For this review, take the finished solid that the model builds, in its own axes (mm). Round coordinates to 2 decimals unless told otherwise and drop trailing zeros. Loops run counter-clockwise (first coordinate to the right, second up) from the corner with the lowest first, then second, coordinate; pieces in that order, holes last. Notation, with made-up numbers: (-13, -7.5) -> (42, -7.5) arc R16 ccw to (42, 11.5) -> close; hole circle Ø9 at (86.5, -24). An arc over 180 degrees is marked (long way). One line per question, with ' | ' between items. Start each with the question number.
1. Consider section A-A (x = -5). Write out the cut boundary in (y, z) (3 decimals).
2. Wall thickness on line 1 along Y through (x, z) = (23, 0.9); line 2 along Y through (x, z) = (36, 1.2) (3 decimals): over which ranges is each line inside the solid? List them lowest first.
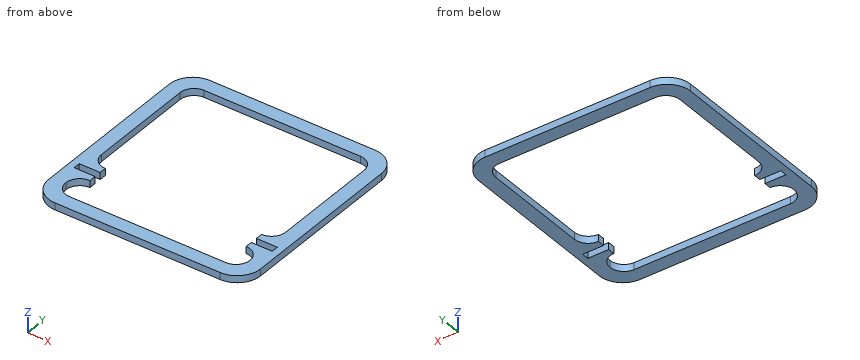
```python
from build123d import *

# Parameters (mm, degrees)
SKETCH1_W           = 96.52
SKETCH1_H           = 96.52
BOSS_EXTRUDE1_DEPTH = 3.175
FILLET1_R           = 10.668
FILLET2_R           = 6.35
FILLET3_R           = 6.35


with BuildPart() as part:
    # Sketch1 → Boss-Extrude1 (new body)
    with BuildSketch(Plane.XY):
        Rectangle(SKETCH1_W, SKETCH1_H)
        Polygon((-41.91, -41.91), (-41.91, -29.21), (-35.56, -29.21), (-35.56, -26.035), (-45.085, -26.035), (-45.085, -22.86), (-35.56, -22.86), (-35.56, -19.685), (-41.91, -19.685), (-41.91, 41.91), (41.91, 41.91), (41.91, -19.685), (35.56, -19.685), (35.56, -22.86), (45.085, -22.86), (45.085, -26.035), (35.56, -26.035), (35.56, -29.21), (41.91, -29.21), (41.91, -41.91), align=None, mode=Mode.SUBTRACT)
    extrude(amount=BOSS_EXTRUDE1_DEPTH)

    # Fillet1
    fillet1_edges = [part.edges().sort_by_distance(p)[0] for p in [
        (48.26, -48.26, 1.5875),
        (-48.26, -48.26, 1.5875),
        (-48.26, 48.26, 1.5875),
        (48.26, 48.26, 1.5875),
    ]]
    fillet(fillet1_edges, radius=FILLET1_R)

    # Fillet2
    fillet2_edges = [part.edges().sort_by_distance(p)[0] for p in [
        (-41.91, -41.91, 1.5875),
        (41.91, -41.91, 1.5875),
        (41.91, 41.91, 1.5875),
        (-41.91, 41.91, 1.5875),
    ]]
    fillet(fillet2_edges, radius=FILLET2_R)

    # Fillet3
    fillet3_edges = [part.edges().sort_by_distance(p)[0] for p in [
        (41.91, -29.21, 1.5875),
        (41.91, -19.685, 1.5875),
        (-41.91, -19.685, 1.5875),
        (-41.91, -29.21, 1.5875),
    ]]
    fillet(fillet3_edges, radius=FILLET3_R - 0.0001)  # a hair under: the kernel refuses the full size


solid = part.part
```
Answer block:
1) outline: (-48.26, 0) -> (-41.91, 0) -> (-41.91, 3.175) -> (-48.26, 3.175) -> close; (41.91, 0) -> (48.26, 0) -> (48.26, 3.175) -> (41.91, 3.175) -> close
2) line 1: y = -48.26 to -41.91, 41.91 to 48.26 | line 2: y = -48.26 to -41.895, -29.225 to -26.035, -22.86 to -19.67, 41.895 to 48.26
